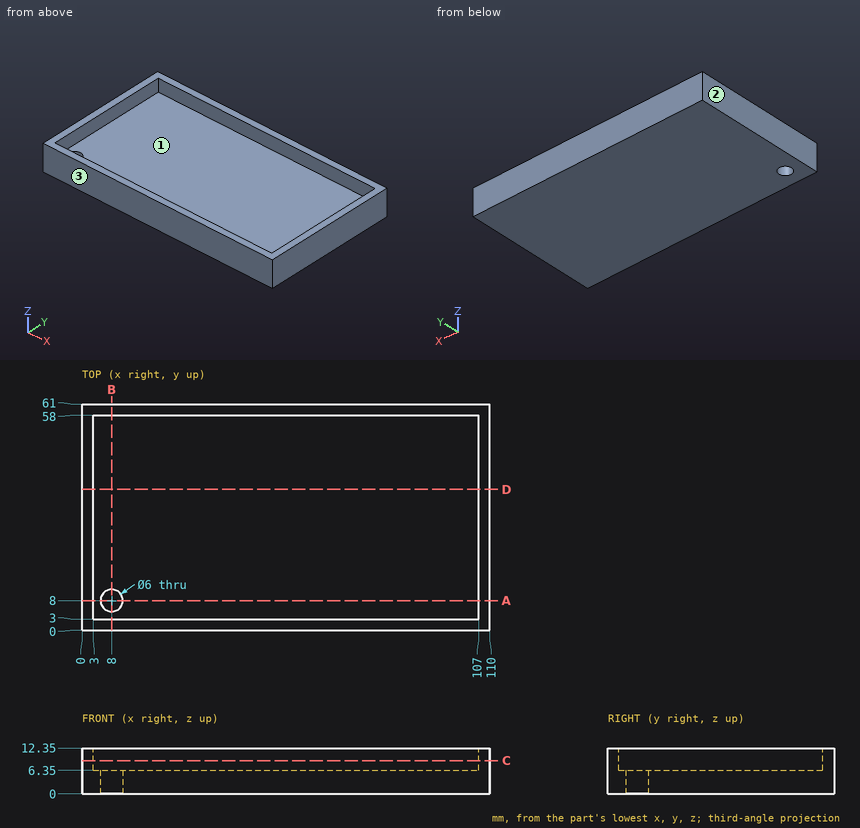
For this review, use the dimensioned drawing (mm, ordinates from the lowest corner) and the shaded views. Give positions to 0.01 mm unless a question says otherwise; leave off trailing zeros. Loops run counter-clockwise (first coordinate to the right, second up) from the corner with the lowest first, then second, coordinate; pieces in that order, holes last. Notation, with made-up numbers: (-16.75, 49) -> (8.25, 49) arc R11 cw to (8.25, 68) -> close; hole circle Ø5 at (-31, 27.25). An arc over 180 degrees is marked (long way). One line per question, with ' | ' between items. Start each with the question number.
(1) For line 1 (Y direction, x = 42.5, z = 11.75); line 2 (Y direction, x = 8, z = 2); line 3 (X direction, y = 30, z = 8.75), list the stretches that pass through material, from the lowest coordinate up.
(2) Draft analysis for pull direction X (two halves, no side actions). For the marked faces 1, 2 and 3, state which applies: +X half, -X half, draft (parallel to the pull), parting line (faces both ways), or undercut.
(3) We need section C-C (z = 9). State the section outline as (x, y) points, and give its area (3 significant figures).
(4) We need section D-D (y = 38). State the section outline as (x, z) points.
(5) We need section B-B (x = 8). State the section outline as (y, z) points.
(6) We need section A-A (y = 8). State the section outline as (x, z) points, and give its area (3 significant figures).
(7) Insertion check: P1, Ø3, axis at x = 56.5, z = 10, coming from the -Y side; P2, Ø12, axis at x = 65.5, y = 45, coming from the +Z side. Each pin has a flat end and moves straight along its axis. Give the tip position at first contact, or say it passes through.
The answers:
1) line 1: y = 0 to 3, 58 to 61 | line 2: y = 0 to 5, 11 to 61 | line 3: x = 0 to 3, 107 to 110
2) face 1: undercut | face 2: -X half | face 3: draft
3) outline: (0, 0) -> (110, 0) -> (110, 61) -> (0, 61) -> close; hole (3, 3) -> (107, 3) -> (107, 58) -> (3, 58) -> close | area: 990 mm^2
4) outline: (0, 0) -> (110, 0) -> (110, 12.35) -> (107, 12.35) -> (107, 6.35) -> (3, 6.35) -> (3, 12.35) -> (0, 12.35) -> close
5) outline: (0, 0) -> (5, 0) -> (5, 6.35) -> (3, 6.35) -> (3, 12.35) -> (0, 12.35) -> close; (11, 0) -> (61, 0) -> (61, 12.35) -> (58, 12.35) -> (58, 6.35) -> (11, 6.35) -> close
6) outline: (0, 0) -> (5, 0) -> (5, 6.35) -> (3, 6.35) -> (3, 12.35) -> (0, 12.35) -> close; (11, 0) -> (110, 0) -> (110, 12.35) -> (107, 12.35) -> (107, 6.35) -> (11, 6.35) -> close | area: 696 mm^2
7) P1: stops at y = 0 | P2: stops at z = 6.35
